Here's how the part is built. I have some questions about the finished solid (model axes, mm). Face numbers are marked on the shaded views. A direction names the side the tool comes from. Coordinates: 2 decimals unless noted, no trailing zeros. Write each loop counter-clockwise with the first axis right and the second up, starting at its lowest first coordinate (ties: lowest second). Pieces come first, ordered by that corner, then holes.
from build123d import *

# Parameters (mm, degrees)
PAD012_DEPTH    = 20
SKETCH024_R     = 2.5
PAD013_DEPTH    = 1
CHAMFER005_SIZE = 2
CHAMFER006_SIZE = 2
CHAMFER007_SIZE = 2.9


with BuildPart() as part:
    # Sketch023 → Pad012 (new body)
    with BuildSketch(Plane.YZ):
        Polygon((0, 0), (0, 70), (-5, 70), (-5, 5), (-65.2, 5), (-65.2, 25), (-70.2, 25), (-70.2, 0), align=None)
    extrude(amount=PAD012_DEPTH)

    # Sketch024 (on Face8 of Pad012) → Pad013 (join)
    with BuildSketch(Plane(origin=(0, 0, 5), x_dir=(0, -1, 0), z_dir=(0, 0, 1))):
        with Locations((35.1, 10)):
            Circle(SKETCH024_R)
    extrude(amount=PAD013_DEPTH)

    # Chamfer005
    chamfer005_edges = [part.edges().sort_by_distance(p)[0] for p in [
        (10, -70.2, 25),
        (20, -70.2, 12.5),
        (0, -70.2, 12.5),
        (10, -70.2, 0),
    ]]
    chamfer(chamfer005_edges, length=CHAMFER005_SIZE)

    # Chamfer006
    chamfer006_edges = [part.edges().sort_by_distance(p)[0] for p in [
        (20, -5, 37.5),
        (10, -5, 70),
        (0, -5, 37.5),
    ]]
    chamfer(chamfer006_edges, length=CHAMFER006_SIZE)

    # Chamfer007
    chamfer007_edges = [part.edges().sort_by_distance(p)[0] for p in [
        (10, -65.2, 25),
    ]]
    chamfer(chamfer007_edges, length=CHAMFER007_SIZE)


solid = part.part
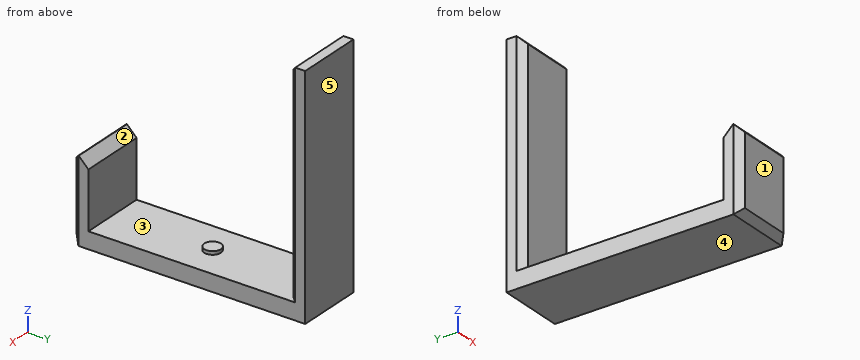
1. I want a section at B-B (y = -35.1). List the corners of the cut face in (x, z) for me, then the cut area to 3 significant figures.
2. On a 3-axis mill with a long thin cutter (end or side, diameter ignored), from which of +Z, -Z, +X, -X, +Y, -Y can I reach the whole of each face in a straight line? I mean the marked faces 1 and 2. Say none if no direction works.
3. I want a section at D-D (z = 53.5). List the corners of the cut face in (x, y) for me.
4. I want a section at C-C (x = 10). List the corners of the cut face in (y, z) for me.
5. For pin 1 Ø2 at (x, z) = (7, 46.5) entering from +Y; pin 2 Ø1 at (x, y) = (15, -35) entering from +Z; pin 3 Ø8 at (x, z) = (12.5, 33) entering from -Y; pin 4 Ø4 at (x, y) = (10, -36) entering from +Z, each with a flat end and sliding along its axis, tell me the tip position at first contact or that it passes through.
6. If I drill on line 1 (Y direction, x = 7.5, z = 21); line 2 (Z direction, x = 3.5, y = -7.5); line 3 (Y direction, x = 11, z = 66.5), over which ranges is the centre line in solid material (lowest first)?
7. I want a section at A-A (z = 7.5). List the corners of the cut face in (x, y) for me.
8. Thinking about a two-plate mould opening in Y: for the marked faces 3, 4 and 5, which applies, pulls with the +Y half, pulls with the -Y half, needs draft (parallel to the pull), parting line crosses it, or undercut?
Response values:
1. outline: (0, 0) - (20, 0) - (20, 5) - (12.5, 5) - (12.5, 6) - (7.5, 6) - (7.5, 5) - (0, 5) - close
1. area: 105 mm2
2. face 1: +Z, -Z, +X, -X, -Y
2. face 2: +Z, +X, -X
3. outline: (0, -3) - (2, -5) - (18, -5) - (20, -3) - (20, 0) - (0, 0) - close
4. outline: (-70.2, 2) - (-68.2, 0) - (0, 0) - (0, 70) - (-3, 70) - (-5, 68) - (-5, 5) - (-32.6, 5) - (-32.6, 6) - (-37.6, 6) - (-37.6, 5) - (-65.2, 5) - (-65.2, 22.1) - (-68.1, 25) - (-68.2, 25) - (-70.2, 23) - close
5. pin 1: stops at y = 0
5. pin 2: stops at z = 5
5. pin 3: stops at y = -5
5. pin 4: stops at z = 6
6. line 1: y = -70.2 to -65.2, -5 to 0
6. line 2: z = 0 to 5
6. line 3: y = -5 to 0
7. outline: (0, -68.2) - (2, -70.2) - (18, -70.2) - (20, -68.2) - (20, -65.2) - (0, -65.2) - close; (0, -3) - (2, -5) - (18, -5) - (20, -3) - (20, 0) - (0, 0) - close
8. face 3: undercut
8. face 4: needs draft
8. face 5: pulls with the +Y half
